Could you check a few things on this drawing? It's one solid part, dimensions in mm from its lowest x, y, z. Coordinates: 2 decimals unless noted, no trailing zeros. Write each loop counter-clockwise with the first axis right and the second up, starting at its lowest first coordinate (ties: lowest second). Pieces come first, ordered by that corner, then holes.
Item 1: I want a section at C-C (z = 1.25). Please give me the cut outline in (x, y), and give its area (3 significant figures).
Item 2: I want a section at B-B (y = 50.5). Please give me the cut outline in (x, z).
Item 3: I want a section at D-D (z = 13.5). Please give me the cut outline in (x, y), and give its area (3 significant figures).
Item 4: Please list where these lines run through material, in increasing order: line 1 (Y direction, x = 12, z = 5.5); line 2 (Z direction, x = 21, y = 52); line 3 (Y direction, x = 12.25, z = 10.75).
Item 5: If we mould it in two halves opening along Y, with no side actions, what happens to the marked faces 1, 2 and 3? For each: pulls with the +Y half, pulls with the -Y half, needs draft (parallel to the pull), parting line crosses it, or undercut.
Item 6: I'm going to push flat-ended pins straight in: P1, Ø6, axis at x = 12, y = 52, coming from the +Z side; P2, Ø1.5, axis at x = 21, z = 6.5, coming from the +Y side; P3, Ø1.5, axis at y = 50.5, z = 9.5, coming from the -X side. Where does each tip first touch, or does it pass through?
Item 7: I want a section at A-A (x = 12). Please give me the cut outline in (y, z).
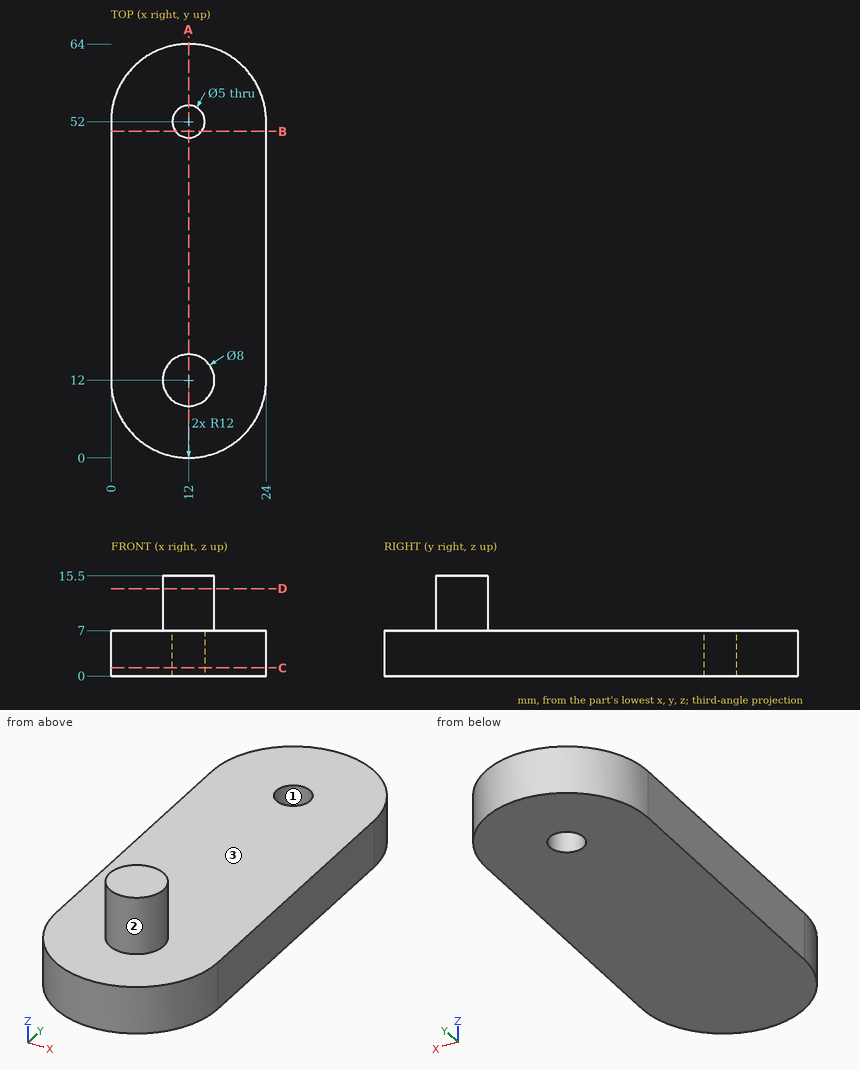
Answer:
1. outline: (0, 12) arc R12 ccw to (24, 12) - (24, 52) arc R12 ccw to (0, 52) - close; hole circle Ø5 at (12, 52)
1. area: 1,390 mm2
2. outline: (0, 0) - (10, 0) - (10, 7) - (0, 7) - close; (14, 0) - (24, 0) - (24, 7) - (14, 7) - close
3. outline: circle Ø8 at (12, 12)
3. area: 50.3 mm2
4. line 1: y = 0 to 49.5, 54.5 to 64
4. line 2: z = 0 to 7
4. line 3: y = 8.01 to 15.99
5. face 1: undercut
5. face 2: parting line crosses it
5. face 3: needs draft
6. P1: stops at z = 7
6. P2: stops at y = 60.71
6. P3: passes through
7. outline: (0, 0) - (49.5, 0) - (49.5, 7) - (16, 7) - (16, 15.5) - (8, 15.5) - (8, 7) - (0, 7) - close; (54.5, 0) - (64, 0) - (64, 7) - (54.5, 7) - close
